Design review of the part shown in the three views and the two pictorial views. Dimensions are in mm from the part's minimum x, y and z. A direction names the side the tool comes from. Round coordinates to 2 decimals unless told otherwise and drop trailing zeros. Order: outer loops, then holes, each group sorted by start corner. A loop starts at its lowest first (then second) coordinate and runs counter-clockwise, first axis right, second up.
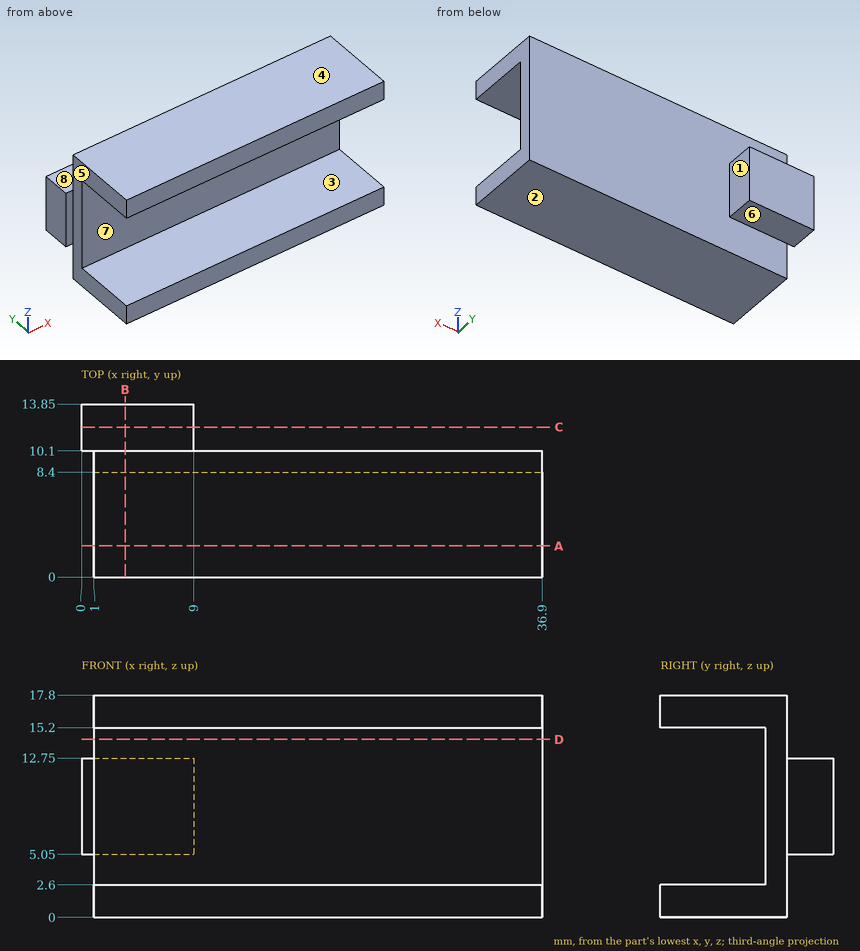
(1) Add section B-B on x = 3.5. Give the boundary of the cut face in (y, z), plus the area to 3 significant figures.
(2) Add section C-C on y = 12. Give the boundary of the cut face in (x, z).
(3) Add section D-D on z = 14.25. Give the boundary of the cut face in (x, y), plus the area to 3 significant figures.
(4) Clearance check with flat-ended pins moving along their axes: P1, Ø6.5, axis at x = 12.5, z = 6.5, coming from the -Y side; P2, Ø1.9, axis at x = 3.5, y = 12.5, coming from the -Z side; P3, Ø5, axis at y = 5.5, z = 10, coming from the -X side; P4, Ø6, axis at y = 5.5, z = 15.5, coming from the -X side. State where each tip first meets the part, or that it passes through.
(5) Add section A-A on y = 2.5. Give the boundary of the cut face in (x, z), plus the area to 3 significant figures.
(6) Wall thickness on L1, parallel to Z at x = 2.5, y = 6.5; L2, parallel to Y at x = 15.5, z = 5; L3, parallel to Y at x = 34.5, z = 2.25: over which ranges is each line inside the solid? List them lowest first.
(7) Tool access review of the marked faces 4, 5, 6, 7 and 8: name each direction out of +Z, -Z, +X, -X, +Y, -Y from which nothing blocks a thin tool from reaching the whole face with its end or side.
(8) Draft analysis for pull direction Z (two halves, no side actions). For the marked faces 1, 2 and 3, state which applies: pulls with the +Z half, pulls with the -Z half, needs draft (parallel to the pull), parting line crosses it, or undercut.
Here are the results:
1. outline: (0, 0) - (10.1, 0) - (10.1, 5.05) - (13.85, 5.05) - (13.85, 12.75) - (10.1, 12.75) - (10.1, 17.8) - (0, 17.8) - (0, 15.2) - (8.4, 15.2) - (8.4, 2.6) - (0, 2.6) - close
1. area: 103 mm2
2. outline: (0, 5.05) - (9, 5.05) - (9, 12.75) - (0, 12.75) - close
3. outline: (1, 8.4) - (36.9, 8.4) - (36.9, 10.1) - (1, 10.1) - close
3. area: 61.0 mm2
4. P1: stops at y = 8.4
4. P2: stops at z = 5.05
4. P3: passes through
4. P4: stops at x = 1
5. outline: (1, 0) - (36.9, 0) - (36.9, 2.6) - (1, 2.6) - close; (1, 15.2) - (36.9, 15.2) - (36.9, 17.8) - (1, 17.8) - close
5. area: 187 mm2
6. L1: z = 0 to 2.6, 15.2 to 17.8
6. L2: y = 8.4 to 10.1
6. L3: y = 0 to 10.1
7. face 4: +Z, +X, -X, +Y, -Y
7. face 5: +Z, -Z, -X, -Y
7. face 6: -Z, +X, -X, +Y
7. face 7: +X, -X, -Y
7. face 8: +Z, +X, -X, +Y
8. face 1: needs draft
8. face 2: pulls with the -Z half
8. face 3: undercut
